Could you check a few things on this model? Use its own coordinates, in mm. Coordinates: 2 decimals unless noted, no trailing zeros. Loops run counter-clockwise (first coordinate to the right, second up) from the corner with the lowest first, then second, coordinate; pieces in that order, holes last.
1) Will these pins go through, and if not, where does the flat tip stop? P1, Ø1.5, axis at x = 17.5, z = -1, coming from the +Y side; P2, Ø9.5, axis at x = -73.5, y = 18.5, coming from the +Z side.
2) Thinking about a two-plate mould opening in Y: for faces 1 (the face through (-31.592, 4.899, -0.022)), 2 (the face through (-76, -8.5, 0)), 3 (the face through (-90.817, 21.007, -0.022)), which applies, released by +Y, released by -Y, zero draft, split by the parting line, or undercut?
3) Imagine slicing it at D-D on x = -72.5. Please give me the cut outline in (y, z).
4) Imagine slicing it at C-C on y = 5.5. Please give me the cut outline in (x, z).
5) Imagine slicing it at B-B on x = 33.5. Please give me the cut outline in (y, z), plus the area to 3 significant figures.
6) Imagine slicing it at A-A on z = 0.3. Give the number of separate pieces and of enclosed holes in the cut face, plus the area to 3 significant figures.
7) If I drill on line 1 along X through (y, z) = (21, -1.05); line 2 along Y through (x, z) = (-33.5, 0.55); line 3 along X through (y, z) = (20, 0.4), over which ranges is the centre line in solid material (lowest first)?
Autodesk Inventor part; units mm, degrees
ref_plane "YZ Plane" through (0, 0, 0) normal (1, 0, 0) x (0, 1, 0)
ref_plane "XZ Plane" through (0, 0, 0) normal (0, 1, 0) x (-1, 0, 0)
ref_plane "XY Plane" through (0, 0, 0) normal (0, 0, 1) x (1, 0, 0)
sketch "Sketch1" plane through (0, 0, 0) normal (0, 0, 1) x (1, 0, 0)
  line L0 (-91.5, -8.5) -> (-64, -8.5)
  line L1 (-91.5, 21.5) -> (-91.5, -8.5)
  line L2 (64, -8.5) -> (91.5, -8.5)
  line L3 (91.5, -8.5) -> (91.5, 21.5)
  arc A0 (64, -8.5) -> (-64, -8.5) centre (0, -208.3) ccw
  arc A1 (91.5, 21.5) -> (-91.5, 21.5) centre (0, -208.3) ccw
  circle A2 centre (-77.5, 0) radius 3
  circle A3 centre (77.5, 0) radius 3
  circle A4 centre (-73.5, 18.5) radius 3
  circle A5 centre (73.5, 18.5) radius 3
  line L4 (-33.5, 5.5) -> (33.5, 5.5) construction
  line L5 (33.5, 5.5) -> (33.5, 31.5) construction
  line L6 (33.5, 31.5) -> (-33.5, 31.5) construction
  line L7 (-33.5, 31.5) -> (-33.5, 5.5) construction
  line L8 (-33.5, 5.5) -> (33.5, 31.5) construction
  line L9 (33.5, 5.5) -> (-33.5, 31.5) construction
  circle A6 centre (-33.5, 31.5) radius 2
  circle A7 centre (33.5, 31.5) radius 2
  circle A8 centre (33.5, 5.5) radius 2
  circle A9 centre (-33.5, 5.5) radius 2
  point P0 (0, 0)
  point P1 (0, 18.5)
  point P2 (0, 18.5)
  dimension "d0" = 155
  dimension "d1" = 77.5
  dimension "d2" = 8.5
  dimension "d3" = 27.5
  dimension "d4" = 14
  dimension "d5" = 14
  dimension "d6" = 30
  dimension "d12" = 6
  dimension "d13" = 18.5
  dimension "d14" = 4
  dimension "d15" = 18.5
  dimension "d16" = 4
  dimension "d17" = 67
  dimension "d18" = 26
  dimension "d19" = 4
  dimension "d20" = 10
  dimension "d22" = 40
extrude "Extrusion1" add sketch "Sketch1" along normal mid plane 3.1242
fillet "Fillet1" radius 4 6 edges at (-91.5, -8.5, 0) (-91.5, 21.5, 0) (-64, -8.5, 0) (64, -8.5, 0) (91.5, -8.5, 0) (91.5, 21.5, 0)
properties part number "Y Motor Plate" material "Aluminum 6061"
Filled in:
1. P1: stops at y = 38.48
1. P2: stops at z = 1.56
2. face 1: undercut
2. face 2: released by -Y
2. face 3: released by +Y
3. outline: (-8.5, -1.56) - (15.67, -1.56) - (15.67, 1.56) - (-8.5, 1.56) - close; (21.33, -1.56) - (28.18, -1.56) - (28.18, 1.56) - (21.33, 1.56) - close
4. outline: (-91.5, -1.56) - (-35.5, -1.56) - (-35.5, 1.56) - (-91.5, 1.56) - close; (-31.5, -1.56) - (31.5, -1.56) - (31.5, 1.56) - (-31.5, 1.56) - close; (35.5, -1.56) - (91.5, -1.56) - (91.5, 1.56) - (35.5, 1.56) - close
5. outline: (-1.19, -1.56) - (3.5, -1.56) - (3.5, 1.56) - (-1.19, 1.56) - close; (7.5, -1.56) - (29.5, -1.56) - (29.5, 1.56) - (7.5, 1.56) - close; (33.5, -1.56) - (36.77, -1.56) - (36.77, 1.56) - (33.5, 1.56) - close
5. area: 93.6 mm2
6. separate pieces: 1
6. enclosed holes: 8
6. area: 6,620 mm2
7. line 1: x = -90.82 to -75.16, -71.84 to 71.84, 75.16 to 90.82
7. line 2: y = -1.19 to 3.5, 7.5 to 29.5, 33.5 to 36.77
7. line 3: x = -91.31 to -76.1, -70.9 to 70.9, 76.1 to 91.31
